Solid Edge part; units mm, degrees
sketch "Sketch1" plane through (0, 0, 0) normal (0, -1, 0) x (1, 0, 0)
  line L0 (-100, -30) -> (100, -30)
  line L1 (100, -30) -> (100, 30)
  line L2 (100, 30) -> (-100, 30)
  line L3 (-100, 30) -> (-100, -30)
  dimension "D1" = 100
  dimension "D2" = 100
extrude "Protrusion1" add sketch "Sketch1" against normal blind 2
sketch "Sketch2" plane through (0, 0, 0) normal (0, -1, 0) x (1, 0, 0)
  line L0 (-39.6222, 11.5432) -> (-48.7647, 28.7907)
  line L1 (-48.7647, 28.7907) -> (-68.9181, 28.7907)
  line L2 (-68.9181, 28.7907) -> (-78.6631, 12.1124)
  line L3 (-78.6631, 12.1124) -> (-65.8971, 12.1124)
  line L4 (-65.8971, 12.1124) -> (-62.8688, 18.0634)
  line L5 (-62.8688, 18.0634) -> (-55.6447, 18.0634)
  line L6 (-55.6447, 18.0634) -> (-51.8394, 12.1124)
  line L7 (-51.8394, 12.1124) -> (-55.6447, 5.4911)
  line L8 (-55.6447, 5.4911) -> (-62.8688, 5.4911)
  line L9 (-62.8688, 5.4911) -> (-62.8688, -5.6236)
  line L10 (-62.8688, -5.6236) -> (-55.2147, -5.6236)
  line L11 (-55.2147, -5.6236) -> (-51.8394, -11.6625)
  line L12 (-51.8394, -11.6625) -> (-55.2147, -18.0171)
  line L13 (-55.2147, -18.0171) -> (-62.8688, -18.0171)
  line L14 (-62.8688, -18.0171) -> (-65.8971, -11.6625)
  line L15 (-65.8971, -11.6625) -> (-78.6631, -11.6625)
  line L16 (-78.6631, -11.6625) -> (-68.9922, -28.7907)
  line L17 (-48.7647, -28.7907) -> (-68.9922, -28.7907)
  line L18 (-48.7647, -28.7907) -> (-39.6222, -12.3974)
  line L19 (-39.6222, -12.3974) -> (-45.6448, 0)
  line L20 (-45.6448, 0) -> (-39.6222, 11.5432)
  line L21 (-29.8239, 28.7907) -> (-39.0136, 11.3404)
  line L22 (-39.0136, 11.3404) -> (-27.2051, 11.3404)
  line L23 (-27.2051, 11.3404) -> (-23.5794, 17.7709)
  line L24 (-23.5794, 17.7709) -> (-16.2069, 17.7709)
  line L25 (-16.2069, 17.7709) -> (-12.7725, 11.3404)
  line L26 (-12.7725, 11.3404) -> (-16.2069, 5.3584)
  line L27 (-16.2069, 5.3584) -> (-23.5794, 5.3584)
  line L28 (-23.5794, 5.3584) -> (-23.5794, -5.3744)
  line L29 (-23.5794, -5.3744) -> (-16.2069, -5.3744)
  line L30 (-16.2069, -5.3744) -> (-12.7725, -11.9215)
  line L31 (-12.7725, -11.9215) -> (-16.2069, -18.0364)
  line L32 (-16.2069, -18.0364) -> (-23.5794, -18.0364)
  line L33 (-23.5794, -18.0364) -> (-27.2051, -11.9215)
  line L34 (-27.2051, -11.9215) -> (-39.0832, -11.9215)
  line L35 (-39.0832, -11.9215) -> (-39.0211, -12.3974)
  line L36 (-39.0211, -12.3974) -> (-29.8416, -28.7907)
  line L37 (-29.8416, -28.7907) -> (-9.9734, -28.7907)
  line L38 (-9.9734, -28.7907) -> (0, -11.7929)
  line L39 (0, -11.7929) -> (-6.8407, 0)
  line L40 (-6.8407, 0) -> (0, 11.8515)
  line L41 (0, 11.8515) -> (-9.9734, 28.7907)
  line L42 (-9.9734, 28.7907) -> (-29.8239, 28.7907)
  line L43 (9.4303, 28.7907) -> (0, 12.3815)
  line L44 (0, 12.3815) -> (0.2872, 11.8515)
  line L45 (0.2872, 11.8515) -> (12.5492, 11.8515)
  line L46 (12.5492, 11.8515) -> (15.7991, 18.0247)
  line L47 (15.7991, 18.0247) -> (23.265, 18.0247)
  line L48 (23.265, 18.0247) -> (26.8369, 11.8515)
  line L49 (26.8369, 11.8515) -> (23.265, 5.318)
  line L50 (23.265, 5.318) -> (15.7991, 5.318)
  line L51 (15.7991, 5.318) -> (15.7991, -5.632)
  line L52 (15.7991, -5.632) -> (23.265, -5.632)
  line L53 (23.265, -5.632) -> (26.7839, -11.7003)
  line L54 (26.7839, -11.7003) -> (23.265, -17.8487)
  line L55 (23.265, -17.8487) -> (15.768, -17.8487)
  line L56 (15.768, -17.8487) -> (12.2913, -11.7003)
  line L57 (0.3007, -11.6312) -> (12.2913, -11.7003)
  line L58 (0, -12.7084) -> (0.3007, -11.6312)
  line L59 (0, -12.7084) -> (9.391, -28.7907)
  line L60 (9.391, -28.7907) -> (29.5768, -28.7907)
  line L61 (29.5768, -28.7907) -> (39.4696, -11.7929)
  line L62 (39.4696, -11.7929) -> (32.5504, 0)
  line L63 (39.014, 12.1809) -> (32.5504, 0)
  line L64 (29.5768, 28.7907) -> (39.014, 12.1809)
  line L65 (29.5768, 28.7907) -> (9.4303, 28.7907)
  line L66 (39.3531, 11.3913) -> (49.0927, 28.7907)
  line L67 (68.964, 28.7907) -> (49.0927, 28.7907)
  line L68 (78.6631, 11.3946) -> (68.964, 28.7907)
  line L69 (55.3829, -28.7907) -> (78.6631, 11.3946)
  line L70 (42.8739, -28.7907) -> (55.3829, -28.7907)
  line L71 (56.0977, -5.4746) -> (42.8739, -28.7907)
  line L72 (49.0927, -5.4746) -> (56.0977, -5.4746)
  line L73 (49.0927, -5.4746) -> (39.3531, 11.3913)
  line L74 (51.7218, 11.7746) -> (55.3868, 5.6144)
  line L75 (55.3868, 5.6144) -> (62.6387, 5.6144)
  line L76 (62.6387, 5.6144) -> (66.3037, 11.7746)
  line L77 (66.3037, 11.7746) -> (62.6387, 17.9349)
  line L78 (62.6387, 17.9349) -> (55.3868, 17.9349)
  line L79 (55.3868, 17.9349) -> (51.7218, 11.7746)
extrude "ExtrudedProtrusion_3" add sketch "Sketch2" along normal blind 3
sketch "Sketch3" plane through (0, 0, 0) normal (0, -1, 0) x (1, 0, 0)
  line L0 (-100, -30) -> (0, -30)
  line L1 (0, -30) -> (0, 30)
  line L2 (0, 30) -> (-100, 30)
  line L3 (-100, 30) -> (-100, -30)
  line L4 (100, -30) -> (100, 30)
  line L5 (100, 30) -> (78.6631, 30)
  line L6 (78.6631, 30) -> (78.6631, -30)
  line L7 (78.6631, -30) -> (100, -30)
extrude "ExtrudedCutout_1" cut sketch "Sketch3" along normal blind 52.8721
sketch "Sketch4" plane through (0, 0, 0) normal (0, -1, 0) x (1, 0, 0)
  line L0 (-100, 30) -> (-100, -30)
  line L1 (-100, -30) -> (0, -30)
  line L2 (0, -30) -> (0, 30)
  line L3 (0, 30) -> (-100, 30)
  line L4 (100, -30) -> (100, 30)
  line L5 (100, 30) -> (78.6631, 30)
  line L6 (78.6631, 30) -> (78.6631, -30)
  line L7 (78.6631, -30) -> (100, -30)
extrude "ExtrudedCutout_2" cut sketch "Sketch4" against normal blind 13.1606
properties part number "BumbleB0910"
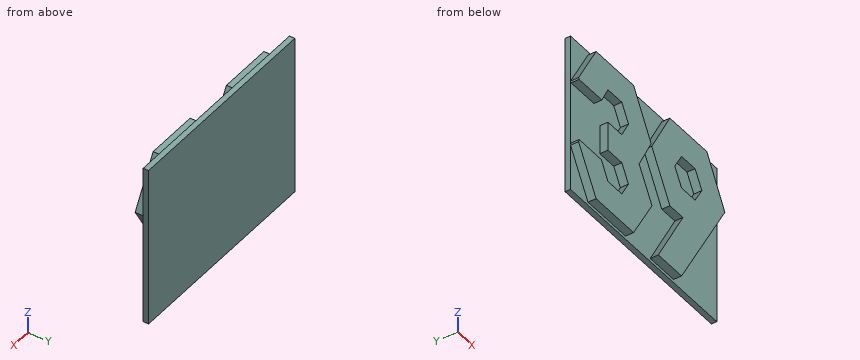
Read the model definition and answer for the solid it produces. Units are mm, in the model's axes. Give positions to 0.01 mm unless a question says otherwise; leave off trailing zeros. Loops run counter-clockwise (first coordinate to the right, second up) from the corner with the lowest first, then second, coordinate; pieces in that order, holes last. Notation, with made-up numbers: (36.5, 68) -> (74.5, 68) arc R7 ccw to (74.5, 72) -> close; hole circle Ø5 at (-13.75, -36.5). An arc over 180 degrees is marked (long way). Use a Markdown table: item, result.
Q1. Section B-B, the plane z = -19.5 is taken. Determine the outline of the cut face in (x, y), then the cut area to 3 significant figures.
Solved:
| item | result |
|---|---|
| outline | (0, 0) -> (3.97, 0) -> (3.97, -3) -> (34.98, -3) -> (34.98, 0) -> (48.14, 0) -> (48.14, -3) -> (60.77, -3) -> (60.77, 0) -> (78.66, 0) -> (78.66, 2) -> (0, 2) -> close |
| area | 288 mm^2 |
Q2. Section A-A, the plane y = -1 is taken. Count the separate pieces of the cut face and the enclosed holes in it, then the cut area to 3 significant figures.
Solved:
| item | result |
|---|---|
| separate pieces | 2 |
| enclosed holes | 1 |
| area | 2,410 mm^2 |
Q3. Find the intervals of material crossed by line 1 along X through (y, z) = (-2.35, -15); line 2 along Z through (x, y) = (53, -2.35); line 3 along Y through (x, z) = (15.5, 7.5), in increasing order.
Solved:
| item | result |
|---|---|
| line 1 | x = 1.34 to 14.16, 24.9 to 37.6, 50.7 to 63.37 |
| line 2 | z = -28.79 to -10.94, -5.47 to 9.63, 13.92 to 28.79 |
| line 3 | y = 0 to 2 |
Q4. Section D-D, the plane z = 14.5 is taken. Determine the outline of the cut face in (x, y).
Solved:
| item | result |
|---|---|
| outline | (0, 0) -> (1.22, 0) -> (1.22, -3) -> (13.94, -3) -> (13.94, 0) -> (25.3, 0) -> (25.3, -3) -> (37.7, -3) -> (37.7, 0) -> (41.09, 0) -> (41.09, -3) -> (53.34, -3) -> (53.34, 0) -> (64.68, 0) -> (64.68, -3) -> (76.93, -3) -> (76.93, 0) -> (78.66, 0) -> (78.66, 2) -> (0, 2) -> close |
Q5. Each of these flat-tipped pins is pushed along its axis until it touches: pin 1 (1.5 mm diameter, centred on x = 59.5, y = -1.5, fed in from -Z); pin 2 (21.5 mm diameter, centred on x = 10.5, z = 6.5, fed in from -Y); pin 3 (0.9 mm diameter, centred on x = 57.5, y = -2, fed in from +Z); pin 4 (1 mm diameter, centred on x = 24.5, y = -2, fed in from -Z). Where does it stop, or does it pass through?
Solved:
| item | result |
|---|---|
| pin 1 | stops at z = -22.98 |
| pin 2 | stops at y = -3 |
| pin 3 | stops at z = 28.79 |
| pin 4 | stops at z = -28.79 |
Q6. Section C-C, the plane x = 58 is taken. Determine the outline of the cut face in (y, z).
Solved:
| item | result |
|---|---|
| outline | (-3, -24.27) -> (0, -24.27) -> (0, -30) -> (2, -30) -> (2, 30) -> (0, 30) -> (0, 28.79) -> (-3, 28.79) -> (-3, 17.93) -> (0, 17.93) -> (0, 5.61) -> (-3, 5.61) -> close |
